from build123d import *

# Parameters (mm, degrees)
F1_DEPTH = 350
F3_DEPTH = 25


with BuildPart() as f1:
    # F0 (on Top) → F1 (new body)
    with BuildSketch(Plane.XY):
        Polygon((0, 7), (0, 0), (7, 0), (7, 5.5), (13, 5.5), (13, 0), (20, 0), (20, 7), (14.5, 7), (14.5, 13), (20, 13), (20, 20), (13, 20), (13, 14.5), (7, 14.5), (7, 20), (0, 20), (0, 13), (5.5, 13), (5.5, 7), align=None)
    extrude(amount=F1_DEPTH)

    # F2 (on face) → F3 (cut)
    with BuildSketch(Plane.XZ):
        with BuildLine():
            ThreePointArc((7, 329.6261364576), (8.4676776723, 329.158202653), (10, 329))
            ThreePointArc((10, 329), (15.3033008589, 331.1966991411), (17.5, 336.5))
            ThreePointArc((17.5, 336.5), (14.1079191813, 342.774950199), (7, 343.3738635424))
            Line((7, 343.3738635424), (7, 329.6261364576))
        make_face()
        with BuildLine():
            ThreePointArc((7, 343.3738635424), (2.5, 336.5), (7, 329.6261364576))
            Line((7, 329.6261364576), (7, 343.3738635424))
        make_face()
        with BuildLine():
            Line((7, 6.6261364576), (7, 20.3738635424))
            ThreePointArc((7, 20.3738635424), (2.5, 13.5), (7, 6.6261364576))
        make_face()
        with BuildLine():
            ThreePointArc((10, 21), (8.4676776723, 20.841797347), (7, 20.3738635424))
            Line((7, 20.3738635424), (7, 6.6261364576))
            ThreePointArc((7, 6.6261364576), (14.1079191813, 7.225049801), (17.5, 13.5))
            ThreePointArc((17.5, 13.5), (15.3033008589, 18.8033008589), (10, 21))
        make_face()
    extrude(amount=-F3_DEPTH, mode=Mode.SUBTRACT)


solid = f1.part
Design review of the part built by this model. Coordinates are the model's own, in mm. A direction names the side the tool comes from. Coordinates: 2 decimals unless noted, no trailing zeros. Order: outer loops, then holes, each group sorted by start corner. A loop starts at its lowest first (then second) coordinate and runs counter-clockwise, first axis right, second up. Notation, with made-up numbers: (53.25, -34.75) -> (71.25, -34.75) arc R17 cw to (71.25, -2.75) -> close; hole circle Ø6 at (63.5, -3). An arc over 180 degrees is marked (long way). Use one line per item in the form item = value. Start each with the question number.
(1) For probe 1 along Y at (x, z) = (2.5, 171); probe 2 along Z at (x, y) = (9, 9.75); probe 3 along Z at (x, y) = (5, 13.75), list the stretches that pass through material, from the lowest coordinate up.
(2) The part is to be moulded in two halves that separate along Y. For faces 1 (the flat face through (17, 7, 173)), 2 (the flat face through (10, 5.5, 347)), 3 (the flat face through (13, 17, 173)), say which applies: +Y half, -Y half, draft (parallel to the pull), parting line (faces both ways), or undercut.
(3) Add section A-A on z = 200.5. State the section outline as (x, y) points.
(4) For faces 4 (the flat face through (5.5, 10, 4)), 5 (the flat face through (10, 14.5, 173)), 6 (the flat face through (13, 3, 173)), 7 (the flat face through (14.5, 10, 4)), list the 3-axis set-ups (+Z, -Z, +X, -X, +Y, -Y) from which the entire face can be reached by the end or side of a thin tool; tool diameter is ignored.
(5) Insertion check: pin 1 (1.8 mm diameter, centred on x = 11, z = 5, fed in from -Y); pin 2 (1.8 mm diameter, centred on x = 10.5, z = 3, fed in from +Y); pin 3 (1.8 mm diameter, centred on y = 9.5, z = 208, fed in from -X). Each pin has a flat end and moves straight along its axis. Give the tip position at first contact, or say it passes through.
Answer block:
q1.probe_1 = 0 to 7, 13 to 20
q1.probe_2 = 0 to 6.07, 20.93 to 329.07, 343.93 to 350
q1.probe_3 = 0 to 7.91, 19.09 to 330.91, 342.09 to 350
q2.face_1 = undercut
q2.face_2 = -Y half
q2.face_3 = draft
q3.outline = (0, 0) -> (7, 0) -> (7, 5.5) -> (13, 5.5) -> (13, 0) -> (20, 0) -> (20, 7) -> (14.5, 7) -> (14.5, 13) -> (20, 13) -> (20, 20) -> (13, 20) -> (13, 14.5) -> (7, 14.5) -> (7, 20) -> (0, 20) -> (0, 13) -> (5.5, 13) -> (5.5, 7) -> (0, 7) -> close
q4.face_4 = +Z, -Z, -X
q4.face_5 = +Z, -Z, +Y
q4.face_6 = +Z, -Z, -Y
q4.face_7 = +Z, -Z, +X
q5.pin_1 = 5.5
q5.pin_2 = 14.5
q5.pin_3 = 5.5
